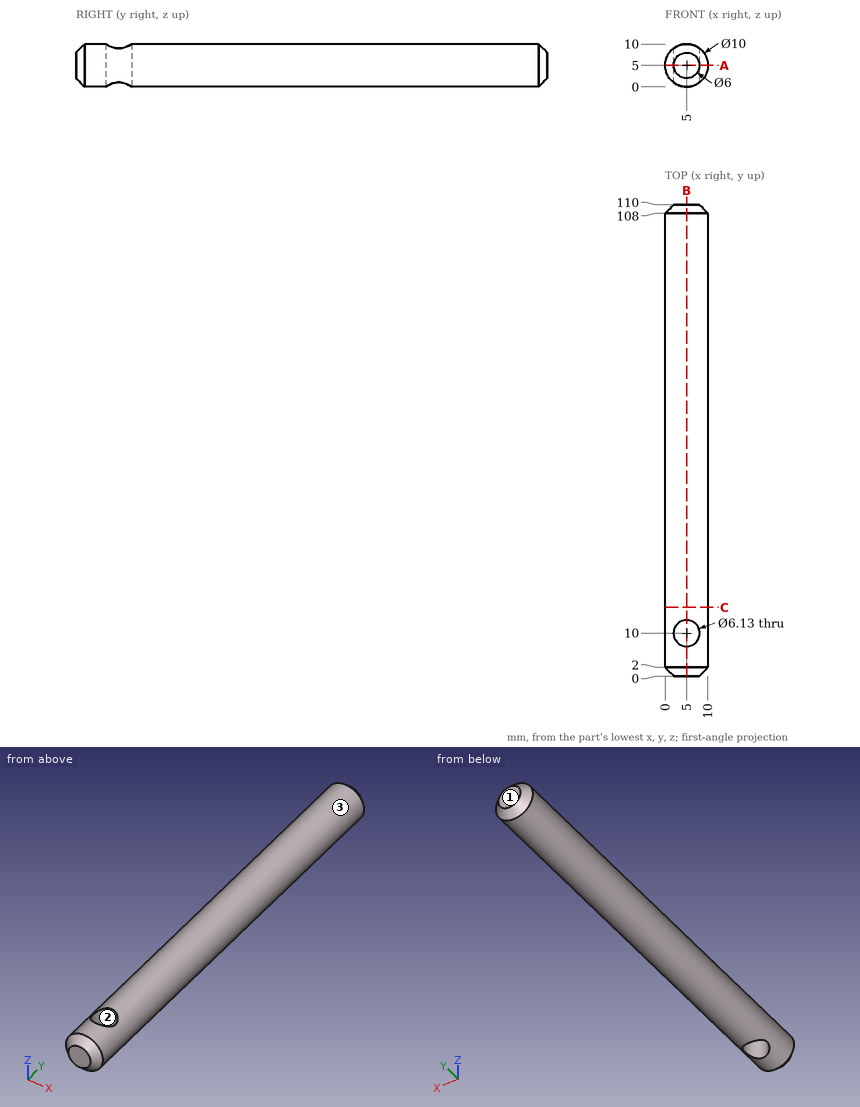
The drawing under review shows one solid part. Ordinate dimensions are in mm from its lowest x, y, z. Coordinates: 2 decimals unless noted, no trailing zeros. Write each loop counter-clockwise with the first axis right and the second up, starting at its lowest first coordinate (ties: lowest second). Pieces come first, ordered by that corner, then holes. Notation, with made-up numbers: (14.25, 87.25) -> (19.25, 87.25) arc R20 cw to (19.25, 107.25) -> close; hole circle Ø3 at (21, 55). An arc over 180 degrees is marked (long way). Write each question's results on one line, items separated by ' | '. Start each with the question number.
1) Consider section A-A (z = 5). Write out the cut boundary in (x, y) (3 decimals).
2) Consider section B-B (x = 5). Write out the cut boundary in (y, z) (3 decimals), plus the area to 3 significant figures.
3) Insertion check: pin 1 (6 mm diameter, centred on x = 3, z = 4.5, fed in from -Y); pin 2 (3 mm diameter, centred on x = 1.5, y = 16.5, fed in from -Z); pin 3 (2 mm diameter, centred on y = 37.5, z = 8.5, fed in from -X). Each pin has a flat end and moves straight along its axis. Give the tip position at first contact, or say it passes through.
4) Wall thickness on L1, parallel to Y at x = 5, z = 7 (3 decimals); L2, parallel to X at y = 10, z = 5.25 (3 decimals); L3, parallel to Z at x = 9, y = 41: over which ranges is each line inside the solid? List them lowest first. Write a range as [from, to].
5) The part is to be moulded in two halves that separate along X. For the marked faces 1, 2 and 3, say which applies: +X half, -X half, draft (parallel to the pull), parting line (faces both ways), or undercut.
6) Consider section C-C (y = 16). Write out the cut boundary in (x, z), plus the area to 3 significant figures.
Geometry says:
1) outline: (0, 2) -> (2, 0) -> (8, 0) -> (10, 2) -> (10, 108) -> (8, 110) -> (2, 110) -> (0, 108) -> close; hole circle Ø6.13 at (5, 10)
2) outline: (0, 2) -> (2, 0) -> (6.935, 0) -> (6.935, 10) -> (2, 10) -> (0, 8) -> close; (13.065, 0) -> (108, 0) -> (110, 2) -> (110, 8) -> (108, 10) -> (13.065, 10) -> close | area: 1,030 mm^2
3) pin 1: y = 0 | pin 2: z = 0.42 | pin 3: x = 0.67
4) L1: [0, 6.935], [13.065, 110] | L2: [0.006, 1.935], [8.065, 9.994] | L3: [2, 8]
5) face 1: draft | face 2: undercut | face 3: parting line
6) outline: circle Ø10 at (5, 5) | area: 78.5 mm^2
